```python
from build123d import *

# Parameters (mm, degrees)
F0_W     = 59
F0_H     = 50
F0_R     = 7.5
F1_DEPTH = 4
F2_W     = 4
F2_H     = 50
F3_DEPTH = 63


with BuildPart() as f1:
    # F0 (on Top) → F1 (new body)
    with BuildSketch(Plane.XY):
        Rectangle(F0_W, F0_H)
        Circle(F0_R, mode=Mode.SUBTRACT)
    extrude(amount=F1_DEPTH)

    # F2 (on face) → F3 (join)
    with BuildSketch(Plane(origin=(0, 0, 0), x_dir=(1, 0, 0), z_dir=(0, 0, -1))):
        with Locations((-31.5, 0)):
            Rectangle(F2_W, F2_H)
    extrude(amount=-F3_DEPTH)


solid = f1.part
```
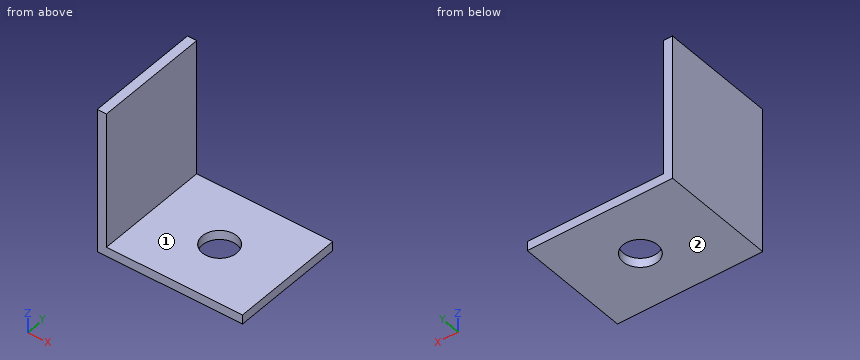
The model under review builds one solid part; all positions refer to its coordinate system, in mm. Face numbers are marked on the shaded views. A direction names the side the tool comes from. Give positions to 0.01 mm unless a question says otherwise; leave off trailing zeros. Write each loop counter-clockwise with the first axis right and the second up, starting at its lowest first coordinate (ties: lowest second). Pieces come first, ordered by that corner, then holes. Notation, with made-up numbers: (74.5, -22) - (79.5, -22) arc R37 ccw to (79.5, 16) - close; hole circle Ø2 at (9.5, 74.5). An arc over 180 degrees is marked (long way). Answer in a Markdown table with one row per item. Add a question column.
1. We need section A-A on y = 0. Write out the cut boundary in (x, z).
2. Tool access review of the marked faces 1 and 2: name each direction out of +Z, -Z, +X, -X, +Y, -Y from which nothing blocks a thin tool from reaching the whole face with its end or side.
3. Wall thickness on line 1 along Y through (x, z) = (0, 2.05); line 2 along Z through (x, y) = (16.5, -21); line 3 along X through (y, z) = (13.5, 15): over which ranges is each line inside the solid? List them lowest first. Write a range as [from, to].
4. We need section B-B on x = 0. Write out the cut boundary in (y, z), then the cut area to 3 significant figures.
5. Insertion check: P1, Ø1.5, axis at y = 0, z = 42, coming from the +X side; P2, Ø10, axis at x = 19.5, y = 1, coming from the +Z side. Each pin has a flat end and moves straight along its axis. Give the tip position at first contact, or say it passes through.
6. We need section C-C on z = 21.5. Write out the cut boundary in (x, y).
7. We need section D-D on y = 22. Write out the cut boundary in (x, z), then the cut area to 3 significant figures.
Ans:
| question | item | result |
|---|---|---|
| 1 | outline | (-33.5, 0) - (-7.5, 0) - (-7.5, 4) - (-29.5, 4) - (-29.5, 63) - (-33.5, 63) - close; (7.5, 0) - (29.5, 0) - (29.5, 4) - (7.5, 4) - close |
| 2 | face 1 | +Z, +X, +Y, -Y |
| 2 | face 2 | -Z, +X, -X, +Y, -Y |
| 3 | line 1 | y = [-25, -7.5], [7.5, 25] |
| 3 | line 2 | z = [0, 4] |
| 3 | line 3 | x = [-33.5, -29.5] |
| 4 | outline | (-25, 0) - (-7.5, 0) - (-7.5, 4) - (-25, 4) - close; (7.5, 0) - (25, 0) - (25, 4) - (7.5, 4) - close |
| 4 | area | 140 mm^2 |
| 5 | P1 | stops at x = -29.5 |
| 5 | P2 | stops at z = 4 |
| 6 | outline | (-33.5, -25) - (-29.5, -25) - (-29.5, 25) - (-33.5, 25) - close |
| 7 | outline | (-33.5, 0) - (29.5, 0) - (29.5, 4) - (-29.5, 4) - (-29.5, 63) - (-33.5, 63) - close |
| 7 | area | 488 mm^2 |
